```python
from build123d import *

# Parameters (mm, degrees)
SKETCH1_W           = 41.91
SKETCH1_H           = 44.45
BOSS_EXTRUDE1_DEPTH = 4.2926
FILLET1_R           = 2.54
SKETCH2_W           = 4.2926
SKETCH2_H           = 25.4
SKETCH2_W_2         = 8.636
SKETCH2_H_2         = 12.7
CUT_EXTRUDE2_DEPTH  = 4.2926
FILLET3_R           = 1.27


with BuildPart() as part:
    # Sketch1 → Boss-Extrude1 (new body)
    with BuildSketch(Plane.XY):
        Rectangle(SKETCH1_W, SKETCH1_H)
    extrude(amount=BOSS_EXTRUDE1_DEPTH)

    # Fillet1
    fillet1_edges = [part.edges().sort_by_distance(p)[0] for p in [
        (20.955, -22.225, 2.1463),
        (-20.955, -22.225, 2.1463),
        (-20.955, 22.225, 2.1463),
        (20.955, 22.225, 2.1463),
    ]]
    fillet(fillet1_edges, radius=FILLET1_R)

    # Sketch2 → Cut-Extrude2 (cut)
    with BuildSketch(Plane.XY.offset(4.2926)):
        with Locations((-11.4173, 9.525)):
            Rectangle(SKETCH2_W, SKETCH2_H)
        with Locations((11.4173, 9.525)):
            Rectangle(SKETCH2_W, SKETCH2_H)
        with Locations((0, -15.875)):
            Rectangle(SKETCH2_W_2, SKETCH2_H_2)
    extrude(amount=-CUT_EXTRUDE2_DEPTH, mode=Mode.SUBTRACT)

    # Fillet3
    fillet3_edges = [part.edges().sort_by_distance(p)[0] for p in [
        (-9.271, 22.225, 2.1463),
        (9.271, 22.225, 2.1463),
    ]]
    fillet(fillet3_edges, radius=FILLET3_R)


solid = part.part
```
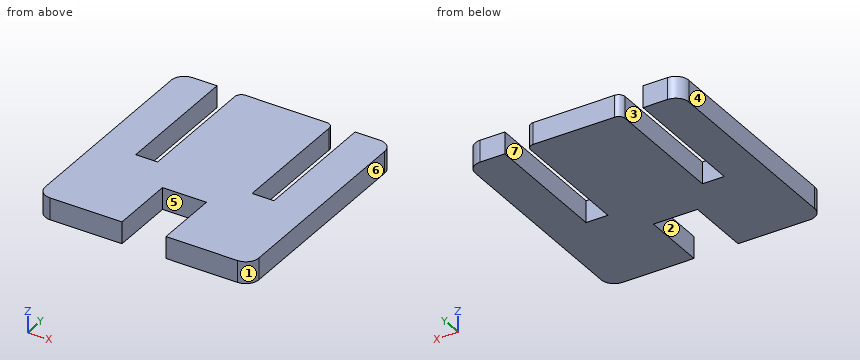
Model file for the job. Use its own axes, mm. Face numbers are marked on the shaded views. A direction names the side the tool comes from. Round coordinates to 2 decimals unless told otherwise and drop trailing zeros. Write each loop counter-clockwise with the first axis right and the second up, starting at its lowest first coordinate (ties: lowest second). Pieces come first, ordered by that corner, then holes. Notation, with made-up numbers: (43, -9.5) -> (91, -9.5) arc R11 ccw to (91, 0.5) -> close; hole circle Ø10 at (55.5, -20.75). An arc over 180 degrees is marked (long way). Answer as CSV lines item,"result".
1. Slice it at A-A, the plane y = -15.5. List the corners of the cut face in (x, z) (3 decimals).
Resolved:
outline,"(-20.955, 0) -> (-4.318, 0) -> (-4.318, 4.293) -> (-20.955, 4.293) -> close; (4.318, 0) -> (20.955, 0) -> (20.955, 4.293) -> (4.318, 4.293) -> close"
2. Slice it at C-C, the plane y = 6.5. List the corners of the cut face in (x, z) (3 decimals), plus the area to 3 significant figures.
Resolved:
outline,"(-20.955, 0) -> (-13.564, 0) -> (-13.564, 4.293) -> (-20.955, 4.293) -> close; (-9.271, 0) -> (9.271, 0) -> (9.271, 4.293) -> (-9.271, 4.293) -> close; (13.564, 0) -> (20.955, 0) -> (20.955, 4.293) -> (13.564, 4.293) -> close"
area,"143 mm²"
3. Slice it at B-B, the plane z = 2.85. List the corners of the cut face in (x, y) (3 decimals), plus the area to 3 significant figures.
Resolved:
outline,"(-20.955, -19.685) arc R2.54 ccw to (-18.415, -22.225) -> (-4.318, -22.225) -> (-4.318, -9.525) -> (4.318, -9.525) -> (4.318, -22.225) -> (18.415, -22.225) arc R2.54 ccw to (20.955, -19.685) -> (20.955, 19.685) arc R2.54 ccw to (18.415, 22.225) -> (13.564, 22.225) -> (13.564, -3.175) -> (9.271, -3.175) -> (9.271, 20.955) arc R1.27 ccw to (8.001, 22.225) -> (-8.001, 22.225) arc R1.27 ccw to (-9.271, 20.955) -> (-9.271, -3.175) -> (-13.564, -3.175) -> (-13.564, 22.225) -> (-18.415, 22.225) arc R2.54 ccw to (-20.955, 19.685) -> close"
area,"1,530 mm²"
4. Tool access for the marked faces 5, 6 and 7: list every direction of +Z, -Z, +X, -X, +Y, -Y with a clear straight run to the whole face (end or side of a thin tool).
Resolved:
face 5,"+Z, -Z, -Y"
face 6,"+Z, -Z, +X, +Y, -Y"
face 7,"+Z, -Z, +Y"
5. Slice it at D-D, the plane x = -1. List the corners of the cut face in (y, z) (3 decimals), plus the area to 3 significant figures.
Resolved:
outline,"(-9.525, 0) -> (22.225, 0) -> (22.225, 4.293) -> (-9.525, 4.293) -> close"
area,"136 mm²"
6. Pin check, flat tip, straight feed: pin 1 Ø2 at (x, z) = (11, 2.5) entering from +Y (3 decimals). Stop position of the tip, or through.
Resolved:
pin 1,"y = -3.175"
7. Mould opens along X. For the marked faces 1, 2, 3 and 4 say: +X half, -X half, draft (parallel to the pull), parting line (faces both ways), or undercut.
Resolved:
face 1,"+X half"
face 2,"undercut"
face 3,"undercut"
face 4,"-X half"
8. Drill centre lines: line 1 (X direction, y = 3, z = 2) (3 decimals); line 2 (X direction, y = -13, z = 2.75) (3 decimals); line 3 (Y direction, x = -10, z = 2.1) (3 decimals). Where is each one in solid material? Low to high.
Resolved:
line 1,"-20.955 to -13.564, -9.271 to 9.271, 13.564 to 20.955"
line 2,"-20.955 to -4.318, 4.318 to 20.955"
line 3,"-22.225 to -3.175"
